Model file for the job. Use its own axes, mm. Give positions to 0.01 mm unless a question says otherwise; leave off trailing zeros. Loops run counter-clockwise (first coordinate to the right, second up) from the corner with the lowest first, then second, coordinate; pieces in that order, holes last. Notation, with made-up numbers: M 79.25,21 L 136.25,21 A17 ccw 136.25,29 Z; hole C 2.5,50 d2. An arc over 180 degrees is marked long. Answer in a Markdown table with one row per item.
```python
from build123d import *

# Parameters (mm, degrees)
SKETCH1_R                = 6
SKETCH1_R_2              = 3
SKETCH1_W                = 70
SKETCH1_H                = 7.937253934
SKETCH1_R_3              = 2
BOSS_EXTRUDE1_DEPTH      = 3
SKETCH2_R                = 6
SKETCH2_R_2              = 3
BOSS_EXTRUDE2_DEPTH      = 5
BOSS_EXTRUDE2_DEPTH_BACK = 8


with BuildPart() as part:
    # Sketch1 → Boss-Extrude1 (new body)
    with BuildSketch(Plane.XY):
        Circle(SKETCH1_R)
        Circle(SKETCH1_R_2, mode=Mode.SUBTRACT)
        with Locations((39.5, 0)):
            Rectangle(SKETCH1_W, SKETCH1_H)
        with Locations((70, 0)):
            Circle(SKETCH1_R_3, mode=Mode.SUBTRACT)
    extrude(amount=BOSS_EXTRUDE1_DEPTH)

    # Sketch2 → Boss-Extrude2 (add, two sides)
    with BuildSketch(Plane.XY.offset(3)) as boss_extrude2_sk:
        Circle(SKETCH2_R)
        Circle(SKETCH2_R_2, mode=Mode.SUBTRACT)
    extrude(amount=BOSS_EXTRUDE2_DEPTH)
    extrude(boss_extrude2_sk.sketch, amount=-BOSS_EXTRUDE2_DEPTH_BACK)


solid = part.part
```
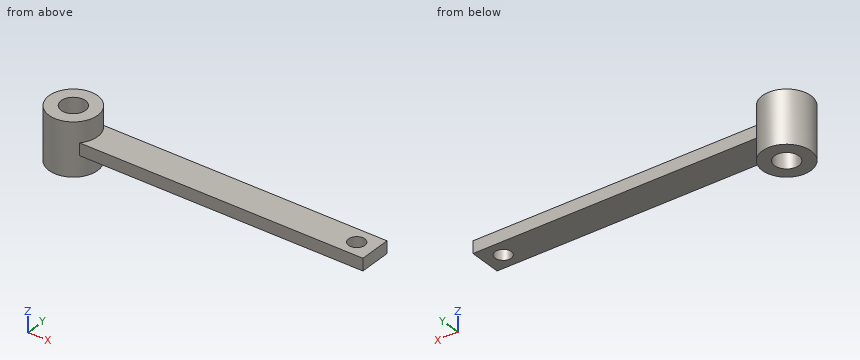
Q1. Saw through at A-A (x = 70). Give the cut face in (y, z), and give its area (3 significant figures).
Reported:
| item | result |
|---|---|
| outline | M -3.97,0 L -2,0 L -2,3 L -3.97,3 Z; M 2,0 L 3.97,0 L 3.97,3 L 2,3 Z |
| area | 11.8 mm² |
Q2. Saw through at C-C (y = 0). Give the cut face in (x, z), and give its area (4 significant figures).
Reported:
| item | result |
|---|---|
| outline | M -6,-5 L -3,-5 L -3,8 L -6,8 Z; M 3,-5 L 6,-5 L 6,0 L 68,0 L 68,3 L 6,3 L 6,8 L 3,8 Z; M 72,0 L 74.5,0 L 74.5,3 L 72,3 Z |
| area | 271.5 mm² |
Q3. Probe probe 1 along Y at (x, z) = (0, 1.05); probe 2 along Y at (x, z) = (70, 2.45); probe 3 along Z at (x, y) = (46, 3). List the from-to ranges inside material, lowest first.
Reported:
| item | result |
|---|---|
| probe 1 | -6 to -3, 3 to 6 |
| probe 2 | -3.97 to -2, 2 to 3.97 |
| probe 3 | 0 to 3 |
Q4. Drop flat-ended pins along their axis: pin 1 (3 mm diameter, centred on y = -0.5, z = -3, fed in from +X); pin 2 (3.5 mm diameter, centred on x = 26.5, z = 1, fed in from -Y); pin 3 (1.5 mm diameter, centred on x = 14, y = -4.5, fed in from +Z); pin 4 (3.5 mm diameter, centred on x = 0, y = 0, fed in from -Z). Give the stop position or say it passes through.
Reported:
| item | result |
|---|---|
| pin 1 | x = 6 |
| pin 2 | y = -3.97 |
| pin 3 | z = 3 |
| pin 4 | through |
Q5. Saw through at D-D (x = 0). Give the cut face in (y, z), and give its area (3 significant figures).
Reported:
| item | result |
|---|---|
| outline | M -6,-5 L -3,-5 L -3,8 L -6,8 Z; M 3,-5 L 6,-5 L 6,8 L 3,8 Z |
| area | 78.0 mm² |
Q6. Saw through at B-B (z = 2). Give the cut face in (x, y), and give its area (3 significant figures).
Reported:
| item | result |
|---|---|
| outline | M 4.5,-3.97 L 74.5,-3.97 L 74.5,3.97 L 4.5,3.97 A6 ccw long Z; hole C 0,0 d6; hole C 70,0 d4 |
| area | 620 mm² |
